```python
from build123d import *

# Parameters (mm, degrees)
SKETCH1_W                              = 240.03
SKETCH1_H                              = 360.68
BOSS_EXTRUDE1_DEPTH                    = 12.446
TAP_DRILL_FOR_M10_HELICOIL1_AT_2_COUNT = 2
TAP_DRILL_FOR_M10_HELICOIL1_AT_2_PITCH = 63.5


with BuildPart() as part:
    # Sketch1 → Boss-Extrude1 (new body)
    with BuildSketch(Plane(origin=(0, 0, 0), x_dir=(1, 0, 0), z_dir=(0, 1, 0))):
        Rectangle(SKETCH1_W, SKETCH1_H)
    extrude(amount=BOSS_EXTRUDE1_DEPTH)

    # Sketch4 → Tap Drill for M10 Helicoil1 (revolve, cut)
    with BuildSketch(Plane(origin=(80.01, 12.446, -51.435), x_dir=(0, 0, 1), z_dir=(1, 0, 0))):
        Polygon((0, 0), (0, 28.15451905), (5.25, 25.0000008), (5.25, 0), align=None)
    tap_drill_for_m10_helicoil1 = revolve(axis=Axis((80.01, 18.796, -51.435), (0, -1, 0)), mode=Mode.SUBTRACT)

    # Tap Drill for M10 Helicoil1 at 2: Tap Drill for M10 Helicoil1 ×2
    with Locations(*[(0, 0, i * TAP_DRILL_FOR_M10_HELICOIL1_AT_2_PITCH) for i in range(1, TAP_DRILL_FOR_M10_HELICOIL1_AT_2_COUNT)]):
        add(tap_drill_for_m10_helicoil1, mode=Mode.SUBTRACT)

    # Mirror1: Tap Drill for M10 Helicoil1 across plane
    add(tap_drill_for_m10_helicoil1.mirror(Plane.ZY), mode=Mode.SUBTRACT)

    # Mirror1 copy 1 sketch → Mirror1 copy 1 (revolve, cut)
    with BuildSketch(Plane(origin=(-80.01, 12.446, 12.065), x_dir=(0, 0, 1), z_dir=(-1, 0, 0))):
        Polygon((0, 0), (0, -28.15451905), (5.25, -25.0000008), (5.25, 0), align=None)
    revolve(axis=Axis((-80.01, 18.796, 12.065), (0, 1, 0)), mode=Mode.SUBTRACT)


solid = part.part
```
Source: CAD feature listing. Evaluate the final solid. Frame: model axes, mm. Round coordinates to 2 decimals unless told otherwise and drop trailing zeros. Loops run counter-clockwise (first coordinate to the right, second up) from the corner with the lowest first, then second, coordinate; pieces in that order, holes last. Notation, with made-up numbers: M 51,-24.75 L 58,-24.75 A22 cw 58,12.25 Z; hole C 61,3 d1. An arc over 180 degrees is marked long. Use a Markdown table: item, result. Add a question column.
1. Section query A-A on x = 80.01. Return the cut outline in (y, z) (3 decimals).
2. Contact query for a flat-ended pin moving along its axis: P1, Ø9.5, axis at x = 80.01, z = 12.065, coming from the +Y side. Output: stop coordinate, or through.
3. Mould query, pull axis Z, two halves, no side actions, for faces 1 (the flat face through (-2, 6, -180.34)), 2 (the flat face through (-120.015, 6, 3)), 3 (the cylindrical face through (-74.805, 6.31, 11.382)). Classes: pulls with the +Z half, pulls with the -Z half, needs draft (parallel to the pull), parting line crosses it, or undercut.
4. Line query: line 1 (X direction, y = 11.25, z = 13) (3 decimals); line 2 (Z direction, x = 80.01, y = 9.25) (3 decimals); line 3 (Z direction, x = -83, y = 8.75). Output: solid intervals per line, ascending.
Reported:
| question | item | result |
|---|---|---|
| 1 | outline | M 0,-180.34 L 12.446,-180.34 L 12.446,-56.685 L 0,-56.685 Z; M 0,-46.185 L 12.446,-46.185 L 12.446,6.815 L 0,6.815 Z; M 0,17.315 L 12.446,17.315 L 12.446,180.34 L 0,180.34 Z |
| 2 | P1 | passes through |
| 3 | face 1 | pulls with the -Z half |
| 3 | face 2 | needs draft |
| 3 | face 3 | undercut |
| 4 | line 1 | x = -120.015 to -85.176, -74.844 to 74.844, 85.176 to 120.015 |
| 4 | line 2 | z = -180.34 to -56.685, -46.185 to 6.815, 17.315 to 180.34 |
| 4 | line 3 | z = -180.34 to -55.75, -47.12 to 7.75, 16.38 to 180.34 |
